from build123d import *

# Parameters (mm, degrees)
POCKET_DEPTH = 6


with BuildPart() as part:
    # Sketch → Revolution (revolve)
    with BuildSketch(Plane.XY):
        with BuildLine():
            Line((6, 0), (9, 0))
            Line((9, 0), (9, -10.8))
            ThreePointArc((7.8, -12), (8.648528, -11.648528), (9, -10.8))
            Line((7.8, -12), (0, -12))
            Line((0, -12), (0, 20))
            Line((0, 20), (4.925, 20))
            Line((4.925, 20), (6, 19.379348))
            Line((6, 19.379348), (6, 0))
        make_face()
    revolve(axis=Axis((0, 0, 0), (0, 1, 0)))

    # Sketch001 → Pocket (cut)
    with BuildSketch(Plane.XZ.offset(12)):
        Polygon((-5, 2.886751), (-5, -2.886751), (0, -5.773503), (5, -2.886751), (5, 2.886751), (0, 5.773503), align=None)
    extrude(amount=-POCKET_DEPTH, mode=Mode.SUBTRACT)


solid = part.part
Input: part model. Units: mm. Frame: model coordinates. A direction names the side the tool comes from. Coordinates: 2 decimals unless noted, no trailing zeros. Order: outer loops, then holes, each group sorted by start corner. A loop starts at its lowest first (then second) coordinate and runs counter-clockwise, first axis right, second up. Notation, with made-up numbers: M 81,43.5 L 87,43.5 A29 ccw 87,68.5 Z; hole C 1.25,83.5 d10. An arc over 180 degrees is marked long. Write item = value, one per line. Start each with the question number.
(1) Pull-direction query (Z, two-part tool) for faces 4 (the cylindrical face through (-1.172, -5.476, -8.923)), 5 (the flat face through (2, -12, 5)), 6 (the flat face through (2.465, -9.042, -4.35)); classes: released by +Z, released by -Z, zero draft, split by the parting line, or undercut.
(2) Section C-C on y = 12.5. Output: boundary loops of the cut face in (x, z).
(3) Line query: line 1 along Y through (x, z) = (-2.5, 2.25); line 2 along Z through (x, y) = (0, 5); line 3 along Y through (x, z) = (-5.5, 2.75). Output: solid intervals per line, ascending. Write a range as [from, to].
(4) Reachability of faces 1 (the flat face through (5, -9, 0)), 2 (the cylindrical face through (-6, 10, 0)), 3 (the flat face through (0, 20, 0)) from +Z, -Z, +X, -X, +Y, -Y: full face, straight path, thin tool, end or side. Return the list, or none.
(5) Section A-A on z = 0. Output: boundary loops of the cut face in (x, y) (3 decimals), and give its area (3 significant figures).
(6) Section B-B on y = -7.5. Output: boundary loops of the cut face in (x, z), and give its area (3 significant figures).
(7) First-contact query: P1, Ø5, axis at x = -0.5, z = 2.5, coming from the -Y side; P2, Ø8, axis at y = 13, z = -1, coming from the -X side; P3, Ø1, axis at x = 6.5, y = -2, coming from the -Z side. Flat tips, straight axial feed; report the tip coordinate or a pass-through.
Result set:
q1.face_4 = split by the parting line
q1.face_5 = zero draft
q1.face_6 = undercut
q2.outline = C 0,0 d12
q3.line_1 = [-6, 20]
q3.line_2 = [-6, 6]
q3.line_3 = [-12, 0]
q4.face_1 = -Y
q4.face_2 = +Y
q4.face_3 = +Z, -Z, +X, -X, +Y
q5.outline = M -9,-10.8 A1.2 ccw -7.8,-12 L -5,-12 L -5,-6 L 5,-6 L 5,-12 L 7.8,-12 A1.2 ccw 9,-10.8 L 9,0 L 6,0 L 6,19.379 L 4.925,20 L -4.925,20 L -6,19.379 L -6,0 L -9,0 Z
q5.area = 395 mm²
q6.outline = C 0,0 d18; hole M -5,-2.89 L 0,-5.77 L 5,-2.89 L 5,2.89 L 0,5.77 L -5,2.89 Z
q6.area = 168 mm²
q7.P1 = -6
q7.P2 = -6
q7.P3 = -6.71
